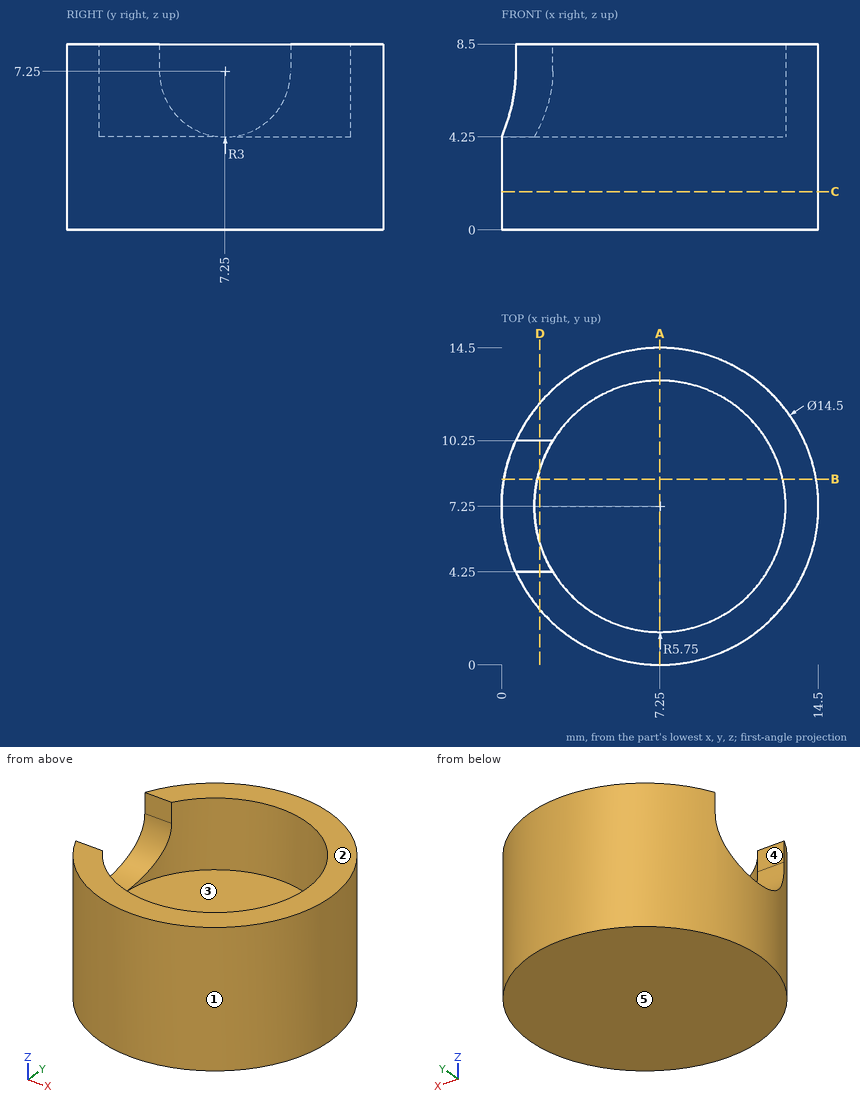
The drawing under review shows one solid part. Ordinate dimensions are in mm from its lowest x, y, z. A direction names the side the tool comes from. Give positions to 0.01 mm unless a question says otherwise; leave off trailing zeros. Write each loop counter-clockwise with the first axis right and the second up, starting at its lowest first coordinate (ties: lowest second). Pieces come first, ordered by that corner, then holes. Notation, with made-up numbers: (6, 29) -> (56, 29) arc R27 cw to (56, 45) -> close; hole circle Ø6 at (7, -29.75). An arc over 180 degrees is marked (long way). Put each result on its own line as item: value.
(1) We need section C-C, the plane z = 1.75. Give the boundary of the cut face in (x, y), and give its area (3 significant figures).
Results are:
outline: circle Ø14.5 at (7.25, 7.25)
area: 165 mm²
(2) The part is to be moulded in two halves that separate along X. For the marked faces 1, 2 and 3, say which applies: pulls with the +X half, pulls with the -X half, needs draft (parallel to the pull), parting line crosses it, or undercut.
Results are:
face 1: parting line crosses it
face 2: needs draft
face 3: undercut
(3) To check wall thickness, follow probe 1 along Z at (x, y) = (10.25, 6.5); probe 2 along Y at (x, z) = (9.5, 4.75); probe 3 along Y at (x, z) = (1.5, 6.5). State the ranges of each line that lie inside material, in increasing order. Write a range as from..to.
Results are:
probe 1: 0..4.25
probe 2: 0.36..1.96, 12.54..14.14
probe 3: 2.83..4.35, 10.15..11.67
(4) We need section B-B, the plane y = 8.5. Give the boundary of the cut face in (x, z).
Results are:
outline: (0.11, 0) -> (14.39, 0) -> (14.39, 8.5) -> (12.86, 8.5) -> (12.86, 4.25) -> (1.64, 4.25) -> (1.64, 4.52) -> (0.11, 4.52) -> close
(5) For pin 1 Ø1 at (x, z) = (1, 7.5) entering from +Y; pin 2 Ø1 at (x, z) = (2.5, 5.5) entering from -Y; pin 3 Ø4 at (x, z) = (12.5, 4) entering from -Y, all flat-tipped, find the tip position at first contact; note any pin that passes through.
Results are:
pin 1: y = 11.67
pin 2: y = 1.38
pin 3: y = 0.77
(6) We need section D-D, the plane x = 1.75. Give the boundary of the cut face in (y, z), and give its area (3 significant figures).
Results are:
outline: (2.53, 0) -> (11.97, 0) -> (11.97, 8.5) -> (10.25, 8.5) -> (10.25, 7.25) arc R3 cw to (8.93, 4.76) -> (8.93, 4.25) -> (5.57, 4.25) -> (5.57, 4.76) arc R3 cw to (4.25, 7.25) -> (4.25, 8.5) -> (2.53, 8.5) -> close
area: 58.1 mm²
(7) Tool access review of the marked faces 4 and 5: name each direction out of +Z, -Z, +X, -X, +Y, -Y from which nothing blocks a thin tool from reaching the whole face with its end or side.
Results are:
face 4: +Z, -X
face 5: -Z, +X, -X, +Y, -Y
(8) We need section A-A, the plane x = 7.25. Give the boundary of the cut face in (y, z), and give its area (3 significant figures).
Results are:
outline: (0, 0) -> (14.5, 0) -> (14.5, 8.5) -> (13, 8.5) -> (13, 4.25) -> (1.5, 4.25) -> (1.5, 8.5) -> (0, 8.5) -> close
area: 74.4 mm²
